Check sheet for the drawn part. Datum: minimum x, y, z corner. Units: mm. A direction names the side the tool comes from. Coordinates: 2 decimals unless noted, no trailing zeros. Write each loop counter-clockwise with the first axis right and the second up, starting at its lowest first coordinate (ties: lowest second). Pieces come first, ordered by that corner, then holes. Notation, with made-up numbers: M -18,48 L 41,48 A21 ccw 41,74 Z; hole C 72,57 d9. An arc over 180 degrees is marked long. Answer as CSV lines item,"result". Start each with the question number.
Q1. Sectioned sample at B-B, the plane x = 123. Record the cut outline in (y, z) (1 decimal).
Q2. Mould release check, pull along X, two halves, no side actions. Record for the marked faces 1 and 2: pulls with the +X half, pulls with the -X half, needs draft (parallel to the pull), parting line crosses it, or undercut.
Q3. Depth check by flat-ended pin: pin 1 Ø3 at (y, z) = (12.5, 9) entering from +X (1 decimal); pin 2 Ø4 at (x, y) = (55.5, 39.5) entering from -Z (1 decimal); pin 3 Ø5 at (x, y) = (125.5, 42) entering from -Z (1 decimal); pin 4 Ø5 at (x, z) = (142.43, 9.53) entering from -Y. Enter the tip coordinate at first touch or a pass-through.
Q4. Thickness scan on line 1 along X through (y, z) = (43, 9) (1 decimal); line 2 along Z through (x, y) = (154, 39) (1 decimal); line 3 along X through (y, z) = (39.5, 10.5) (1 decimal). Record the ranges inside material, lowest first. Write a range as from..to.
Q5. Sectioned sample at A-A, the plane y = 4. Count the separate pieces of the cut face and the enclosed holes in it, then the cut area to 3 significant figures.
Q6. Access from +Z, -Z, +X, -X, +Y, -Y to the whole of each face (thin tool, end or side, straight path). Record for the marked faces 3, 4 and 5.
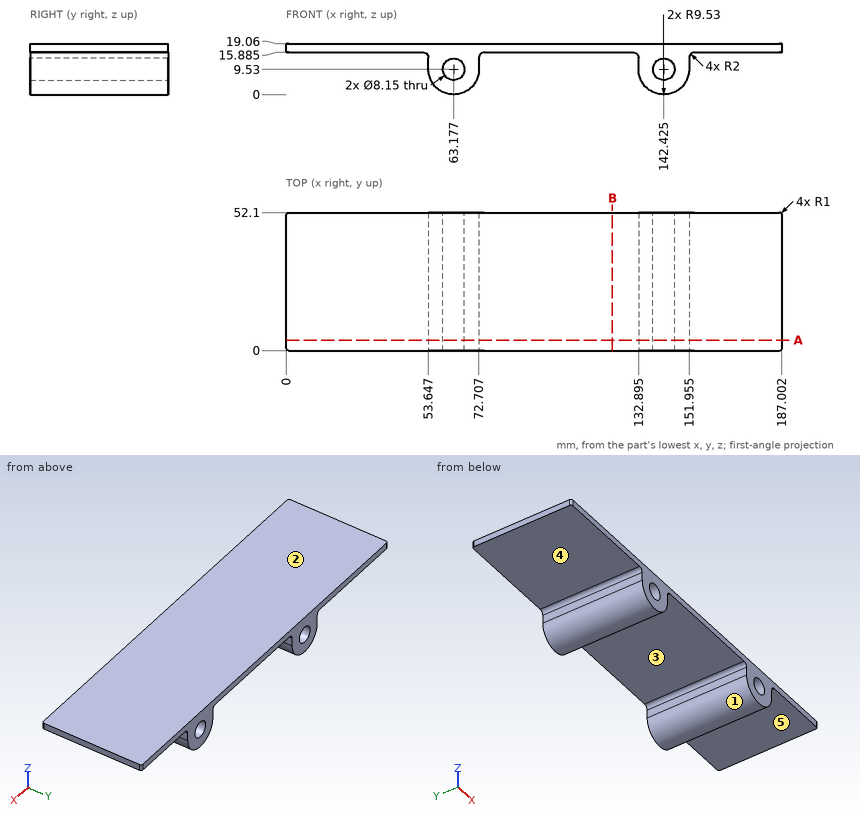
Output:
1,outline,"M 0,15.9 L 52.1,15.9 L 52.1,19.1 L 0,19.1 Z"
2,face 1,"undercut"
2,face 2,"needs draft"
3,pin 1,"stops at x = 152"
3,pin 2,"stops at z = 1.9"
3,pin 3,"stops at z = 15.9"
3,pin 4,"passes through"
4,line 1,"x = 53.7..59.1, 67.2..72.7, 132.9..138.4, 146.5..151.9"
4,line 2,"z = 15.9..19.1"
4,line 3,"x = 53.6..59.2, 67.1..72.7, 132.9..138.5, 146.4..152"
5,separate pieces,"1"
5,enclosed holes,"2"
5,area,"1,020 mm^2"
6,face 3,"-Z, +Y, -Y"
6,face 4,"-Z, -X, +Y, -Y"
6,face 5,"-Z, +X, +Y, -Y"
